from build123d import *

# Parameters (mm, degrees)
SKETCH_1_W      = 120
SKETCH_1_H      = 80
EXTRUDE_1_DEPTH = 60
SHELL_1_T       = -5


with BuildPart() as part:
    # Эскиз1 → Бобышка-Вытянуть1 (new body)
    with BuildSketch(Plane(origin=(0, 0, 0), x_dir=(1, 0, 0), z_dir=(0, 1, 0))):
        with Locations((60, 40)):
            Rectangle(SKETCH_1_W, SKETCH_1_H)
    extrude(amount=EXTRUDE_1_DEPTH)

    # Оболочка1
    shell_1_openings = [part.faces().sort_by_distance(p)[0] for p in [
        (60, 0, -40),
    ]]
    offset(amount=SHELL_1_T, openings=shell_1_openings, kind=Kind.INTERSECTION)


solid = part.part
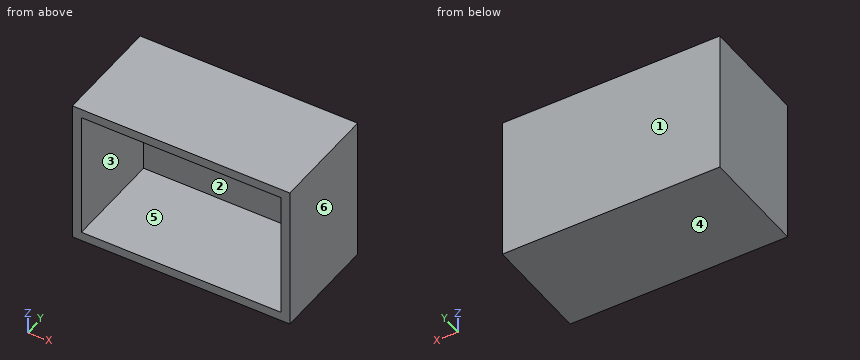
Work out the finished part from the listing and answer in its coordinate system (mm). Face numbers are marked on the shaded views. A direction names the side the tool comes from. Coordinates: 2 decimals unless noted, no trailing zeros. Loops run counter-clockwise (first coordinate to the right, second up) from the corner with the lowest first, then second, coordinate; pieces in that order, holes last. Notation, with made-up numbers: (-32, 77) -> (-16, 77) arc R23 cw to (-16, 89) -> close; hole circle Ø3 at (25.25, 57.25). An arc over 180 degrees is marked (long way). Write each question's results on one line, items separated by ' | '. Start each with the question number.
1) For the marked faces 1 and 2, determine the directions among +Z, -Z, +X, -X, +Y, -Y from which every point of the face is accessible in a straight line to the end or side of a thin tool.
2) Find section A-A on y = 44. Determine the outline of the cut face in (x, z).
3) Find section C-C on x = 49. Determine the outline of the cut face in (y, z), then the cut area to 3 significant figures.
4) Find section B-B on z = -66. Determine the outline of the cut face in (x, y).
5) The mould has two halves that part along Z. Classify the marked faces 3, 4, 5 and 6: pulls with the +Z half, pulls with the -Z half, needs draft (parallel to the pull), parting line crosses it, or undercut.
6) Consider line 1 along Z through (x, y) = (25.5, 14); line 2 along X through (y, z) = (50, -42); line 3 along Y through (x, z) = (96.5, -28.5). Determine where each line is inside the solid, lowest interval first.
Response values:
1) face 1: +Z, -Z, +X, -X, +Y | face 2: -Y
2) outline: (0, -80) -> (120, -80) -> (120, 0) -> (0, 0) -> close; hole (5, -75) -> (115, -75) -> (115, -5) -> (5, -5) -> close
3) outline: (0, -80) -> (60, -80) -> (60, 0) -> (0, 0) -> (0, -5) -> (55, -5) -> (55, -75) -> (0, -75) -> close | area: 950 mm^2
4) outline: (0, 0) -> (5, 0) -> (5, 55) -> (115, 55) -> (115, 0) -> (120, 0) -> (120, 60) -> (0, 60) -> close
5) face 3: undercut | face 4: pulls with the -Z half | face 5: undercut | face 6: needs draft
6) line 1: z = -80 to -75, -5 to 0 | line 2: x = 0 to 5, 115 to 120 | line 3: y = 55 to 60
